CAD build for the part. Positions are in the model's coordinates, mm. A direction names the side the tool comes from. Round coordinates to 2 decimals unless told otherwise and drop trailing zeros. Loops run counter-clockwise (first coordinate to the right, second up) from the corner with the lowest first, then second, coordinate; pieces in that order, holes last.
```python
from build123d import *

# Parameters (mm, degrees)
SKETCH1_W               = 25
SKETCH1_H               = 25
SKETCH1_W_2             = 16.8
SKETCH1_H_2             = 16.8
BOSS_EXTRUDE1_DEPTH     = 50
SKETCH6_W               = 25
SKETCH6_H               = 50
BOSS_EXTRUDE3_DEPTH     = 8
FILLET2_R               = 2
SKETCH7_R               = 4
CUT_EXTRUDE1_DEPTH      = 5
CUT_EXTRUDE4_DEPTH      = 64.73774392
CUT_EXTRUDE4_DEPTH_BACK = 64.73774392
SKETCH8_R               = 2.38125


with BuildPart() as part:
    # Sketch1 → Boss-Extrude1 (new body)
    with BuildSketch(Plane(origin=(0, 0, 0), x_dir=(1, 0, 0), z_dir=(0, 1, 0))):
        Rectangle(SKETCH1_W, SKETCH1_H)
        Rectangle(SKETCH1_W_2, SKETCH1_H_2, mode=Mode.SUBTRACT)
    extrude(amount=BOSS_EXTRUDE1_DEPTH)

    # Sketch6 → Boss-Extrude3 (add)
    with BuildSketch(Plane(origin=(0, 0, 0), x_dir=(1, 0, 0), z_dir=(0, 1, 0))):
        with Locations((0, 12.5)):
            Rectangle(SKETCH6_W, SKETCH6_H)
    extrude(amount=BOSS_EXTRUDE3_DEPTH)

    # Fillet2
    fillet2_edges = [part.edges().sort_by_distance(p)[0] for p in [
        (-12.5, 50, 0),
        (0, 50, 12.5),
        (-12.5, 4, -37.5),
        (-12.5, 8, -25),
        (0, 8, -12.5),
        (12.5, 8, -25),
        (0, 8, -37.5),
        (12.5, 4, -37.5),
        (12.5, 50, 0),
        (12.5, 25, 12.5),
        (-12.5, 25, 12.5),
        (-12.5, 29, -12.5),
        (12.5, 29, -12.5),
        (0, 50, -12.5),
    ]]
    fillet(fillet2_edges, radius=FILLET2_R)

    # Sketch7 → Cut-Extrude1 (cut)
    with BuildSketch(Plane(origin=(0, 8, 0), x_dir=(1, 0, 0), z_dir=(0, 1, 0))):
        with Locations(Location((0, 0, 0), (0, 0, 270))):
            Circle(SKETCH7_R)
        with Locations(Location((0, 25.4, 0), (0, 0, 270))):
            Circle(SKETCH7_R)
    extrude(amount=-CUT_EXTRUDE1_DEPTH, mode=Mode.SUBTRACT)

    # Sketch8 → Cut-Extrude4 (cut, two sides: drawn at the far end of the back side and taken through both)
    with BuildSketch(Plane(origin=(0, 0, 0), x_dir=(1, 0, 0), z_dir=(0, 1, 0)).offset(-CUT_EXTRUDE4_DEPTH_BACK)):
        with Locations(Location((0, 0, 0), (0, 0, 270))):
            Circle(SKETCH8_R)
        with Locations(Location((0, 25.4, 0), (0, 0, 270))):
            Circle(SKETCH8_R)
    extrude(amount=CUT_EXTRUDE4_DEPTH + CUT_EXTRUDE4_DEPTH_BACK, mode=Mode.SUBTRACT)


solid = part.part
```
Item 1: Cut at D-D, the plane z = 0. Give the cut face in (x, y).
Answers follow:
outline: (-12.5, 0) - (-2.38, 0) - (-2.38, 3) - (-4, 3) - (-4, 8) - (-8.4, 8) - (-8.4, 50) - (-10.5, 50) arc R2 ccw to (-12.5, 48) - close; (2.38, 0) - (12.5, 0) - (12.5, 48) arc R2 ccw to (10.5, 50) - (8.4, 50) - (8.4, 8) - (4, 8) - (4, 3) - (2.38, 3) - close
Item 2: Cut at B-B, the plane x = 0. State how many separate pieces and enclosed holes the cut face has, plus the area to 3 significant figures.
Answers follow:
separate pieces: 3
enclosed holes: 0
area: 634 mm2
Item 3: Flat gauge pins, fed straight in: P1, Ø9, axis at x = -2, z = -27.5, coming from the +Y side; P2, Ø1.5, axis at x = -0.5, z = -27.5, coming from the +Y side; P3, Ø1.5, axis at x = 3.5, z = -4, coming from the -Y side; P4, Ø1, axis at x = 0, z = -26.5, coming from the +Y side. Where does each tip first touch, or does it go through?
Answers follow:
P1: stops at y = 8
P2: stops at y = 3
P3: stops at y = 0
P4: passes through
Item 4: 3-axis set-ups, long thin cutter, end or side, ignore diameter. For faces 5 (the flat face through (0, 8, -30)), 6 (the cylindrical face through (11.93, 24.34, 11.9)), 7 (the cylindrical face through (-11.93, 24.34, 11.9)), 8 (the cylindrical face through (11.93, 7.4, -25.15)), 9 (the flat face through (8.4, 29, 0)): which of +Z, -Z, +X, -X, +Y, -Y reach the whole face in a straight line?
Answers follow:
face 5: -Z, +X, -X, +Y
face 6: +Z, +X, +Y, -Y
face 7: +Z, -X, +Y, -Y
face 8: -Z, +X, +Y
face 9: +Y
Item 5: Cut at C-C, the plane y = 46. Give the cut face in (x, z), plus the area to 3 significant figures.
Answers follow:
outline: (-12.5, -10.5) arc R2 ccw to (-10.5, -12.5) - (10.5, -12.5) arc R2 ccw to (12.5, -10.5) - (12.5, 10.5) arc R2 ccw to (10.5, 12.5) - (-10.5, 12.5) arc R2 ccw to (-12.5, 10.5) - close; hole (-8.4, -8.4) - (8.4, -8.4) - (8.4, 8.4) - (-8.4, 8.4) - close
area: 339 mm2
Item 6: Probe line 1 (Z direction, x = -6.25, y = 39); line 2 (X direction, y = 5, z = 0). List the from-to ranges inside material, lowest first.
Answers follow:
line 1: z = -12.5 to -8.4, 8.4 to 12.5
line 2: x = -12.5 to -4, 4 to 12.5
Item 7: Cut at A-A, the plane z = -25.4. Give the cut face in (x, y), plus the area to 3 significant figures.
Answers follow:
outline: (-12.5, 0) - (-2.38, 0) - (-2.38, 3) - (-4, 3) - (-4, 8) - (-10.5, 8) arc R2 ccw to (-12.5, 6) - close; (2.38, 0) - (12.5, 0) - (12.5, 6) arc R2 ccw to (10.5, 8) - (4, 8) - (4, 3) - (2.38, 3) - close
area: 144 mm2
Item 8: Two-plate mould, pull along X, no slides. Class faces 1 (the flat face through (0, 3, -37.5)), 2 (the flat face through (0, 29, 8.4)), 3 (the cylindrical face through (-1.45, 1.48, -1.89)), 4 (the cylindrical face through (11.93, 49.4, -0.15)): released by +X, released by -X, zero draft, split by the parting line, or undercut.
Answers follow:
face 1: zero draft
face 2: undercut
face 3: undercut
face 4: released by +X
